Autodesk Inventor part; units mm, degrees
ref_plane "Arbeitsebene1" through (0, 0, 260) normal (0, 0, 1) x (1, 0, 0)
ref_plane "YZ Plane" through (0, 0, 0) normal (1, 0, 0) x (0, 1, 0)
ref_plane "XZ Plane" through (0, 0, 0) normal (0, 1, 0) x (-1, 0, 0)
sketch "Skizze1" plane through (0, 0, 0) normal (0, 0, 1) x (1, 0, 0)
  line L0 (0, 0) -> (10, 0)
  line L1 (10, 0) -> (10, 10)
  line L2 (10, 10) -> (0, 10)
  line L3 (0, 10) -> (0, 0)
extrude "Extrusion1" add sketch "Skizze1" along normal blind 260
sketch "Skizze2" plane through (0, 0, 0) normal (0, 0, 1) x (1, 0, 0)
  line L0 (0, 0) -> (4, 0)
  line L1 (4, 0) -> (4, 4)
  line L2 (4, 4) -> (0, 4)
  line L3 (0, 4) -> (0, 0)
extrude "Extrusion2" cut sketch "Skizze2" along normal blind 260
sketch "Skizze3" plane through (0, 0, 0) normal (0, 0, 1) x (1, 0, 0)
  line L0 (-3, 6) -> (3, 6)
  line L1 (3, 6) -> (3, 10)
  line L2 (3, 10) -> (-3, 10)
  line L3 (-3, 10) -> (-3, 6)
extrude "Extrusion3" cut sketch "Skizze3" along normal blind 260
sketch "Skizze4" plane through (0, 0, 0) normal (0, 0, 1) x (1, 0, 0)
  line L0 (-3, -10) -> (3, -10)
  line L1 (3, -10) -> (3, -6)
  line L2 (3, -6) -> (-3, -6)
  line L3 (-3, -6) -> (-3, -10)
extrude "Extrusion4" cut sketch "Skizze4" along normal blind 260
sketch "Skizze5" plane through (0, 0, 0) normal (0, 0, 1) x (1, 0, 0)
  line L0 (-10, -3) -> (-6, -3)
  line L1 (-6, -3) -> (-6, 3)
  line L2 (-6, 3) -> (-10, 3)
  line L3 (-10, 3) -> (-10, -3)
extrude "Extrusion5" cut sketch "Skizze5" along normal blind 260
sketch "Skizze6" plane through (0, 0, 0) normal (0, 0, 1) x (1, 0, 0)
  line L0 (6, -3) -> (10, -3)
  line L1 (10, -3) -> (10, 3)
  line L2 (10, 3) -> (6, 3)
  line L3 (6, 3) -> (6, -3)
extrude "Extrusion6" cut sketch "Skizze6" along normal blind 260
ref_plane "Arbeitsebene1" through (0, 0, 260) normal (0, 0, 1) x (1, 0, 0)
sketch "Skizze7" plane through (0, 0, 0) normal (0, 0, 1) x (1, 0, 0)
  circle A0 centre (0, 0) radius 2.5
extrude "Extrusion7" cut sketch "Skizze7" along normal blind 10
sketch "Skizze8" plane through (0, 0, 260) normal (0, 0, 1) x (1, 0, 0)
  circle A0 centre (0, 0) radius 2.5
extrude "Extrusion8" cut sketch "Skizze8" along normal blind 10
properties part number "Aluprofil_20x20_L260"
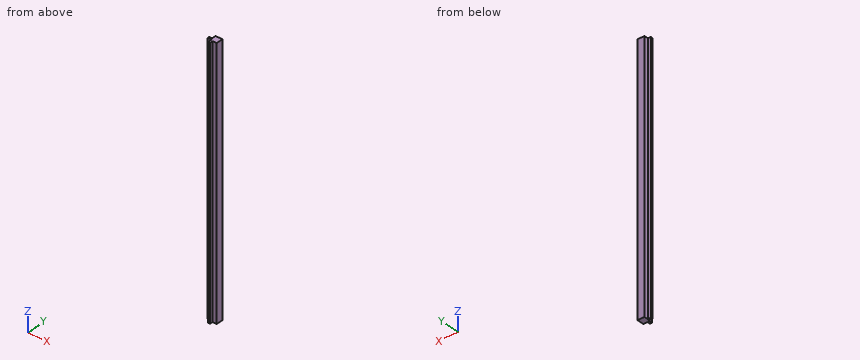
Could you check a few things on this model? Use its own coordinates, in mm. Coordinates: 2 decimals unless noted, no trailing zeros. Order: outer loops, then holes, each group sorted by start corner. A loop starts at its lowest first (then second) coordinate and runs counter-clockwise, first axis right, second up. Notation, with made-up numbers: M -39,84.25 L -4,84.25 A17 ccw -4,109.25 Z; hole C 76,77.5 d11. An arc over 180 degrees is marked long. Use a Markdown table: item, result. Add a question column.
Q1. I want a section at B-B on x = 8.25. List the corners of the cut face in (y, z) for me, then the cut area to 3 significant figures.
Q2. I'm going to push flat-ended pins straight in: pin 1 (4.5 mm diameter, centred on x = 8.5, z = 151.5, fed in from -Y); pin 2 (1.5 mm diameter, centred on y = 1, z = 69.5, fed in from +X); pin 3 (2 mm diameter, centred on y = 2.5, z = 169, fed in from -X). Where does each tip first touch, or does it pass through?
Q3. I want a section at A-A on z = 220. List the corners of the cut face in (x, y) for me.
Q4. If I drill on L1, parallel to Y at x = 6.5, z = 144; L2, parallel to X at y = 2.5, z = 121, over which ranges is the centre line in solid material (lowest first)?
Checked values:
| question | item | result |
|---|---|---|
| 1 | outline | M 3,0 L 10,0 L 10,260 L 3,260 Z |
| 1 | area | 1,820 mm² |
| 2 | pin 1 | y = 3 |
| 2 | pin 2 | x = 6 |
| 2 | pin 3 | x = 4 |
| 3 | outline | M 0,4 L 4,4 L 4,0 L 6,0 L 6,3 L 10,3 L 10,10 L 3,10 L 3,6 L 0,6 Z |
| 4 | L1 | 3 to 10 |
| 4 | L2 | 4 to 6 |
